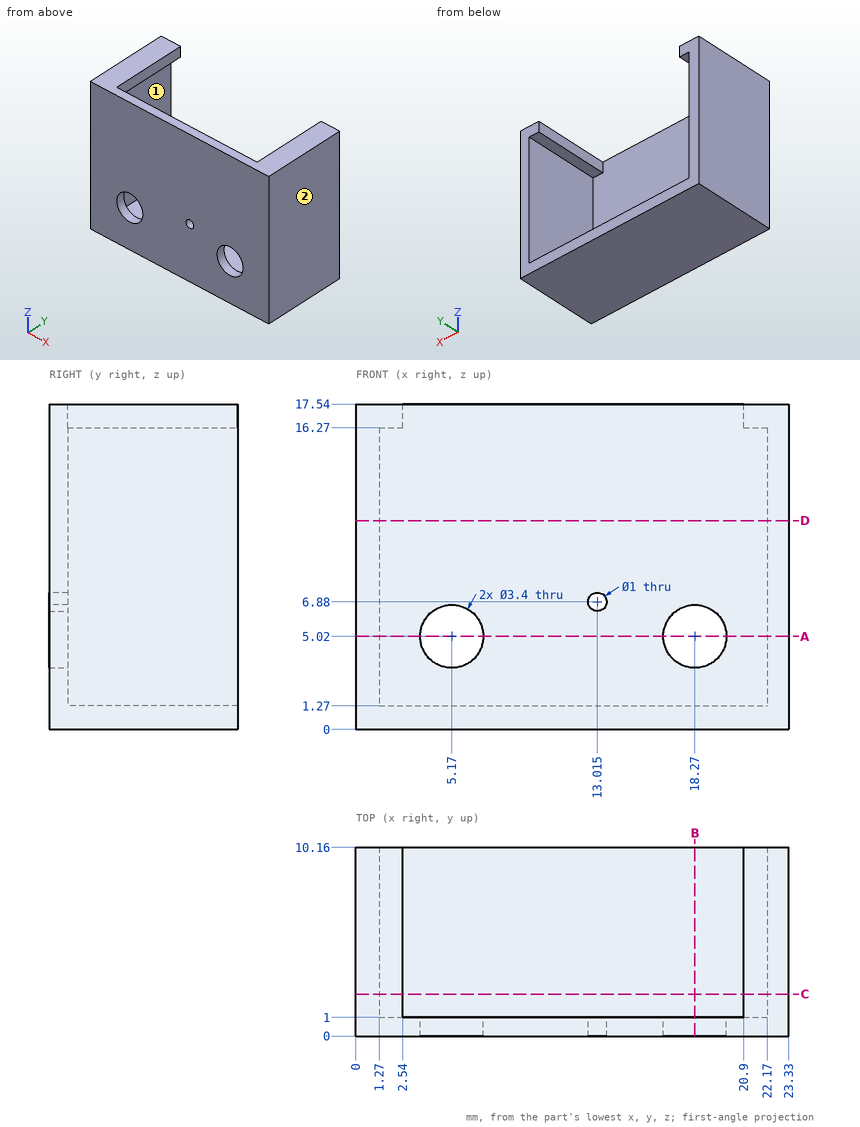
The figure shows three views and two pictorial views of one solid part (mm, origin at its lowest corner). Answer the questions. A direction names the side the tool comes from. Round coordinates to 2 decimals unless told otherwise and drop trailing zeros. Write each loop counter-clockwise with the first axis right and the second up, starting at its lowest first coordinate (ties: lowest second). Pieces come first, ordered by that corner, then holes. Notation, with made-up numbers: (7, -15) -> (42, -15) arc R11 ccw to (42, -5) -> close; hole circle Ø3 at (-13, -25). An arc over 180 degrees is marked (long way). Answer as a JSON object with one key per item and string values. Group by question number.
Q1. Section B-B (x = 18.27) is taken. Write down the section's boundary in (y, z), plus the area to 3 significant figures.
Q2. Section D-D (z = 11.25) is taken. Write down the section's boundary in (x, y), plus the area to 3 significant figures.
Q3. Which of the six approach directions +Z, -Z, +X, -X, +Y, -Y give full straight-line access (tool end or side, diameter ignored) to the marked faces 1 and 2?
Q4. Section A-A (z = 5.02) is taken. Write down the section's boundary in (x, y), plus the area to 3 significant figures.
Q5. Each of these flat-tipped pins is pushed along its axis until it touches: pin 1 Ø2 at (x, y) = (9.5, 3.5) entering from +Z; pin 2 Ø2.5 at (x, z) = (18.27, 5.02) entering from -Y; pin 3 Ø5.5 at (x, z) = (5.17, 5.02) entering from +Y. Where does it stop, or does it pass through?
Q6. Straight lines are drawn through the part: line 1 along X through (y, z) = (0.2, 5.02); line 2 along X through (y, z) = (0.3, 6.88) (3 decimals); line 3 along X through (y, z) = (9, 14.5). For each, find the intervals that lie inside material, in ascending order.
Q7. Section C-C (y = 2.25) is taken. Write down the section's boundary in (x, z), plus the area to 3 significant figures.
Check values:
{
 "1": {"outline": "(0, 0) -> (10.16, 0) -> (10.16, 1.27) -> (1, 1.27) -> (1, 3.32) -> (0, 3.32) -> close; (0, 6.72) -> (1, 6.72) -> (1, 17.54) -> (0, 17.54) -> close", "area": "25.8 mm^2"},
 "2": {"outline": "(0, 0) -> (23.33, 0) -> (23.33, 10.16) -> (22.17, 10.16) -> (22.17, 1) -> (1.27, 1) -> (1.27, 10.16) -> (0, 10.16) -> close", "area": "45.6 mm^2"},
 "3": {"face 1": "+Y", "face 2": "+Z, -Z, +X, +Y, -Y"},
 "4": {"outline": "(0, 0) -> (3.47, 0) -> (3.47, 1) -> (1.27, 1) -> (1.27, 10.16) -> (0, 10.16) -> close; (6.87, 0) -> (16.57, 0) -> (16.57, 1) -> (6.87, 1) -> close; (19.97, 0) -> (23.33, 0) -> (23.33, 10.16) -> (22.17, 10.16) -> (22.17, 1) -> (19.97, 1) -> close", "area": "38.8 mm^2"},
 "5": {"pin 1": "z = 1.27", "pin 2": "through", "pin 3": "y = 1"},
 "6": {"line 1": "0 to 3.47, 6.87 to 16.57, 19.97 to 23.33", "line 2": "0 to 12.515, 13.515 to 23.33", "line 3": "0 to 1.27, 22.17 to 23.33"},
 "7": {"outline": "(0, 0) -> (23.33, 0) -> (23.33, 17.54) -> (20.9, 17.54) -> (20.9, 16.27) -> (22.17, 16.27) -> (22.17, 1.27) -> (1.27, 1.27) -> (1.27, 16.27) -> (2.54, 16.27) -> (2.54, 17.54) -> (0, 17.54) -> close", "area": "72.4 mm^2"}
}
